from build123d import *

# Parameters (mm, degrees)
BOSS_EXTRUDE1_DEPTH = 4
BOSS_EXTRUDE2_DEPTH = 2.5
CHAMFER1_SIZE       = 1
SKETCH4_W           = 6
SKETCH4_H           = 1.5
CUT_EXTRUDE1_DEPTH  = 2.0001
CHAMFER2_SIZE       = 1
SKETCH5_W           = 39.95
SKETCH5_H           = 3.0001
BOSS_EXTRUDE3_DEPTH = 14.1


with BuildPart() as part:
    # Sketch2 → Boss-Extrude1 (new body)
    with BuildSketch(Plane.XY):
        Polygon((-29.9999, -3.0001), (29.9999, -3.0001), (29.9999, -34.771531454), (23.171531454, -41.5999), (-23.171531454, -41.5999), (-29.9999, -34.771531454), align=None)
        Polygon((-28, -33.943145751), (-28, -5), (28, -5), (28, -33.943145751), (22.343145751, -39.6), (-22.343145751, -39.6), align=None, mode=Mode.SUBTRACT)
    extrude(amount=-BOSS_EXTRUDE1_DEPTH)

    # Sketch3 → Boss-Extrude2 (add)
    with BuildSketch(Plane.XY):
        Polygon((-32, 0), (32, 0), (32, -35.6), (24, -43.6), (-24, -43.6), (-32, -35.6), align=None)
    extrude(amount=BOSS_EXTRUDE2_DEPTH)

    # Chamfer1
    chamfer1_edges = [part.edges().sort_by_distance(p)[0] for p in [
        (-32, -17.8, 2.5),
        (-28, -39.6, 2.5),
        (0, -43.6, 2.5),
        (28, -39.6, 2.5),
        (32, -17.8, 2.5),
        (0, 0, 2.5),
    ]]
    chamfer(chamfer1_edges, length=CHAMFER1_SIZE)

    # Sketch4 → Cut-Extrude1 (cut)
    with BuildSketch(Plane.XZ.offset(43.6)):
        Rectangle(SKETCH4_W, SKETCH4_H)
    extrude(amount=-CUT_EXTRUDE1_DEPTH, mode=Mode.SUBTRACT)

    # Chamfer2
    # the kernel refuses this chamfer: 1 mm, written as the material it adds along each edge
    with BuildSketch(Plane(origin=(3, -43.6, 0.75), x_dir=(0.027495876610586487, 0, -0.9996219169112968), z_dir=(0, 1, 0))) as chamfer2_piece_1_section:
        Polygon((CHAMFER2_SIZE * 0.999621916911, CHAMFER2_SIZE * 0.0274958766106), (-CHAMFER2_SIZE * 0.0274958766106, CHAMFER2_SIZE * 0.999621916911), (0, 0), align=None)
    chamfer2_piece_1 = extrude(amount=4.571782988, mode=Mode.PRIVATE)
    chamfer2_piece_1 = split(chamfer2_piece_1, bisect_by=Plane(origin=(2.65, -42.59995, 0), z_dir=(0, 0, 1)), keep=Keep.TOP, mode=Mode.PRIVATE)
    add(chamfer2_piece_1)
    with BuildSketch(Plane(origin=(-3, -43.6, 0.75), x_dir=(-0.027495876610586487, 0, -0.9996219169112968), z_dir=(0, 1, 0))) as chamfer2_piece_2_section:
        Polygon((CHAMFER2_SIZE * 0.999621916911, -CHAMFER2_SIZE * 0.0274958766106), (-CHAMFER2_SIZE * 0.0274958766106, -CHAMFER2_SIZE * 0.999621916911), (0, 0), align=None)
    chamfer2_piece_2 = extrude(amount=4.571782988, mode=Mode.PRIVATE)
    chamfer2_piece_2 = split(chamfer2_piece_2, bisect_by=Plane(origin=(-2.65, -42.59995, 0), z_dir=(0, 0, 1)), keep=Keep.TOP, mode=Mode.PRIVATE)
    add(chamfer2_piece_2)

    # Sketch5 → Boss-Extrude3 (add)
    with BuildSketch(Plane(origin=(0, 0, 0), x_dir=(-1, 0, 0), z_dir=(0, 0, -1))):
        with Locations((0, -1.50005)):
            Rectangle(SKETCH5_W, SKETCH5_H)
    extrude(amount=BOSS_EXTRUDE3_DEPTH)


solid = part.part
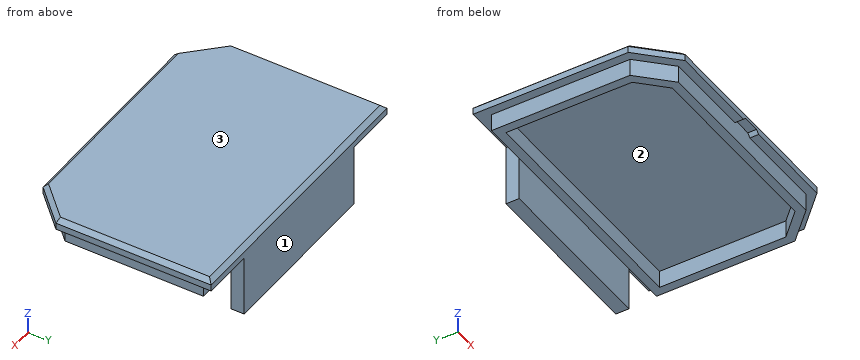
Geometry: final body of the model. Coordinates: model frame, mm. Face numbers are marked on the shaded views. Give positions to 0.01 mm unless a question says otherwise; leave off trailing zeros. Write each loop counter-clockwise with the first axis right and the second up, starting at its lowest first coordinate (ties: lowest second). Pieces come first, ordered by that corner, then holes.
(1) Cut plane C-C, the plane x = 0.5. Return loops of the section in (y, z).
(2) Ray query, line 1 (X direction, y = -6, z = -1.5); line 2 (Y direction, x = 3, z = -2.5); line 3 (Y direction, x = -5, z = -9.25). Return the intervals inside material, ascending.
(3) Cut plane A-A, the plane y = -26. Return loops of the section in (x, z).
(4) Cut plane B-B, the plane z = -2.75. Return loops of the section in (x, y) (3 decimals).
(5) Mould query, pull axis Y, two halves, no side actions, for the marked faces 1, 2 and 3. Classes: released by +Y, released by -Y, zero draft, split by the parting line, or undercut.
(6) Cut plane D-D, the plane z = -6.25. Return loops of the section in (x, y) (3 decimals).
(7) First-contact query: P1, Ø2, axis at y = -20, z = -3, coming from the -X side; P2, Ø8, axis at x = 3.5, y = -29, coming from the -Z side; P3, Ø5, axis at x = 9, z = -11, coming from the -Y side. Flat tips, straight axial feed; report the tip coordinate or a pass-through.
Values follow:
1. outline: (-43.6, 0.75) - (-41.6, 0.75) - (-41.6, -4) - (-39.6, -4) - (-39.6, 0) - (-5, 0) - (-5, -4) - (-3, -4) - (-3, -14.1) - (0, -14.1) - (0, 1.5) - (-1, 2.5) - (-42.6, 2.5) - (-43.6, 1.5) - close
2. line 1: x = -30 to -28, 28 to 30
2. line 2: y = -41.6 to -39.6, -5 to 0
2. line 3: y = -3 to 0
3. outline: (-32, 0) - (-30, 0) - (-30, -4) - (-28, -4) - (-28, 0) - (28, 0) - (28, -4) - (30, -4) - (30, 0) - (32, 0) - (32, 1.5) - (31, 2.5) - (-31, 2.5) - (-32, 1.5) - close
4. outline: (-30, -34.772) - (-23.172, -41.6) - (23.172, -41.6) - (30, -34.772) - (30, -3) - (19.975, -3) - (19.975, 0) - (-19.975, 0) - (-19.975, -3) - (-30, -3) - close; hole (-28, -33.943) - (-22.343, -39.6) - (22.343, -39.6) - (28, -33.943) - (28, -5) - (-28, -5) - close
5. face 1: released by +Y
5. face 2: undercut
5. face 3: zero draft
6. outline: (-19.975, -3) - (19.975, -3) - (19.975, 0) - (-19.975, 0) - close
7. P1: stops at x = -30
7. P2: stops at z = 0
7. P3: stops at y = -3
